For this review, take the finished solid that the model builds, in its own axes (mm). A direction names the side the tool comes from. Round coordinates to 2 decimals unless told otherwise and drop trailing zeros. Write each loop counter-clockwise with the first axis right and the second up, starting at its lowest first coordinate (ties: lowest second). Pieces come first, ordered by that corner, then holes.
from build123d import *

# Parameters (mm, degrees)
SKETCH_4_W          = 0.5
SKETCH_4_H          = 0.5
CUT_EXTRUDE_1_DEPTH = 50


with BuildPart() as part:
    # 草图3 → Revolve 928 (revolve)
    with BuildSketch(Plane.XY, mode=Mode.PRIVATE) as revolve_928_sk:
        with BuildLine():
            Line((0, 0), (17.3, 0))
            Line((17.3, 0), (17.3, 1))
            Line((17.3, 1), (2.1, 1))
            Line((2.1, 1), (1.966, 0.866))
            Line((1.966, 0.866), (1.734, 0.866))
            ThreePointArc((1.734, 0.866), (1.427115657, 0.993115657), (1.3, 1.3))
            Line((1.3, 1.3), (1.3, 2))
            Line((1.3, 2), (0.547706554, 1.934182852))
            ThreePointArc((0.547706554, 1.934182852), (0.157633598, 1.741820158), (0, 1.336466033))
            Line((0, 1.336466033), (0, 0))
        make_face()
    revolve(revolve_928_sk.sketch.rotate(Axis((-2.477021524, 0, 0), (1, 0, 0)), 90), axis=Axis((-2.477021524, 0, 0), (1, 0, 0)))

    # 草图4 → 切除-拉伸1 (cut, symmetric)
    with BuildSketch(Plane.XY):
        with Locations((0.25, 0)):
            Rectangle(SKETCH_4_W, SKETCH_4_H)
    extrude(amount=CUT_EXTRUDE_1_DEPTH, both=True, mode=Mode.SUBTRACT)

    # 草图5 → 切除-旋转1 (revolve, cut)
    with BuildSketch(Plane.XY, mode=Mode.PRIVATE) as cut_revolve_1_sk:
        Polygon((17.097833598, 1), (17.497833598, 1), (17.3, 0.6536), align=None)
    revolve(cut_revolve_1_sk.sketch.rotate(Axis((6.174994867, 0, 0), (-1, 0, 0)), 270), axis=Axis((6.174994867, 0, 0), (-1, 0, 0)), mode=Mode.SUBTRACT)


solid = part.part
(1) For pin 1 Ø1 at (x, y) = (3.5, 1) entering from -Z; pin 2 Ø0.6 at (x, z) = (0.5, 0) entering from -Y, all flat-tipped, find the tip position at first contact; note any pin that passes through.
Geometry check:
pin 1: stops at z = -0.87
pin 2: stops at y = -1.96
(2) We need section C-C, the plane x = 13.5. Give the boundary of the cut face in (y, z).
Geometry check:
outline: circle Ø2 at (0, 0)
(3) For line 1 along X through (y, z) = (0.8, 0.45); line 2 along X through (y, z) = (-0.45, -1.2); line 3 along Z through (x, y) = (12, -0.5), list the stretches that pass through material, from the lowest coordinate up.
Geometry check:
line 1: x = 0 to 1.53, 2.02 to 17.15
line 2: x = 0 to 1.3
line 3: z = -0.87 to 0.87
(4) We need section A-A, the plane z = 0. Give the boundary of the cut face in (x, y).
Geometry check:
outline: (0, -1.34) arc R0.6 ccw to (0.55, -1.93) - (1.3, -2) - (1.3, -1.3) arc R0.43 cw to (1.73, -0.87) - (1.97, -0.87) - (2.1, -1) - (17.1, -1) - (17.3, -0.65) - (17.3, 0.65) - (17.1, 1) - (2.1, 1) - (1.97, 0.87) - (1.73, 0.87) arc R0.43 cw to (1.3, 1.3) - (1.3, 2) - (0.55, 1.93) arc R0.6 ccw to (0, 1.34) - (0, 0.25) - (0.5, 0.25) - (0.5, -0.25) - (0, -0.25) - close
(5) We need section B-B, the plane y = 0. Give the boundary of the cut face in (x, z).
Geometry check:
outline: (0.5, -1.93) arc R0.6 ccw to (0.55, -1.93) - (1.3, -2) - (1.3, -1.3) arc R0.43 cw to (1.73, -0.87) - (1.97, -0.87) - (2.1, -1) - (17.1, -1) - (17.3, -0.65) - (17.3, 0.65) - (17.1, 1) - (2.1, 1) - (1.97, 0.87) - (1.73, 0.87) arc R0.43 cw to (1.3, 1.3) - (1.3, 2) - (0.55, 1.93) arc R0.6 ccw to (0.5, 1.93) - close
(6) For faces 1 (the face through (0, 1, 0)), 2 (the face through (9, 1, 0)), list the 3-axis set-ups (+Z, -Z, +X, -X, +Y, -Y) from which the entire face can be reached by the end or side of a thin tool; tool diameter is ignored.
Geometry check:
face 1: +Z, -Z, -X, +Y, -Y
face 2: +X
